Input: dimensioned drawing with shaded views. Units: mm. Origin: part minimum x, y, z. Give positions to 0.01 mm unless a question says otherwise; leave off trailing zeros. Write each loop counter-clockwise with the first axis right and the second up, starting at its lowest first coordinate (ties: lowest second). Pieces come first, ordered by that corner, then holes. Notation, with made-up numbers: (65.25, 14.25) -> (113.25, 14.25) arc R20 cw to (113.25, 24.25) -> close; hole circle Ø7 at (40.5, 59). An arc over 180 degrees is marked (long way). Answer as a JSON object with one key per item and string values. Group by question number.
(1) Section query A-A on x = 15. Output: boundary loops of the cut face in (y, z), plus the area to 3 significant figures.
(2) Section query B-B on y = 2.5. Output: boundary loops of the cut face in (x, z).
(3) Contact query for flat-ended pins moving along their axis: pin 1 Ø1.5 at (x, y) = (5.5, 0.5) entering from -Z; pin 2 Ø3 at (x, z) = (5, 15) entering from +Y; pin 3 Ø1.5 at (y, z) = (4, 8.5) entering from -X; pin 4 Ø2 at (x, y) = (4.5, 1.5) entering from +Z. Output: stop coordinate, or through.
(4) Material intervals for probe 1 along X at (y, z) = (1.7, 15); probe 2 along X at (y, z) = (1.95, 13.25), sorted ascending.
(5) Draft query along X for the marked faces 1, 2 and 3. Return one class per face: +X half, -X half, draft (parallel to the pull), parting line (faces both ways), or undercut.
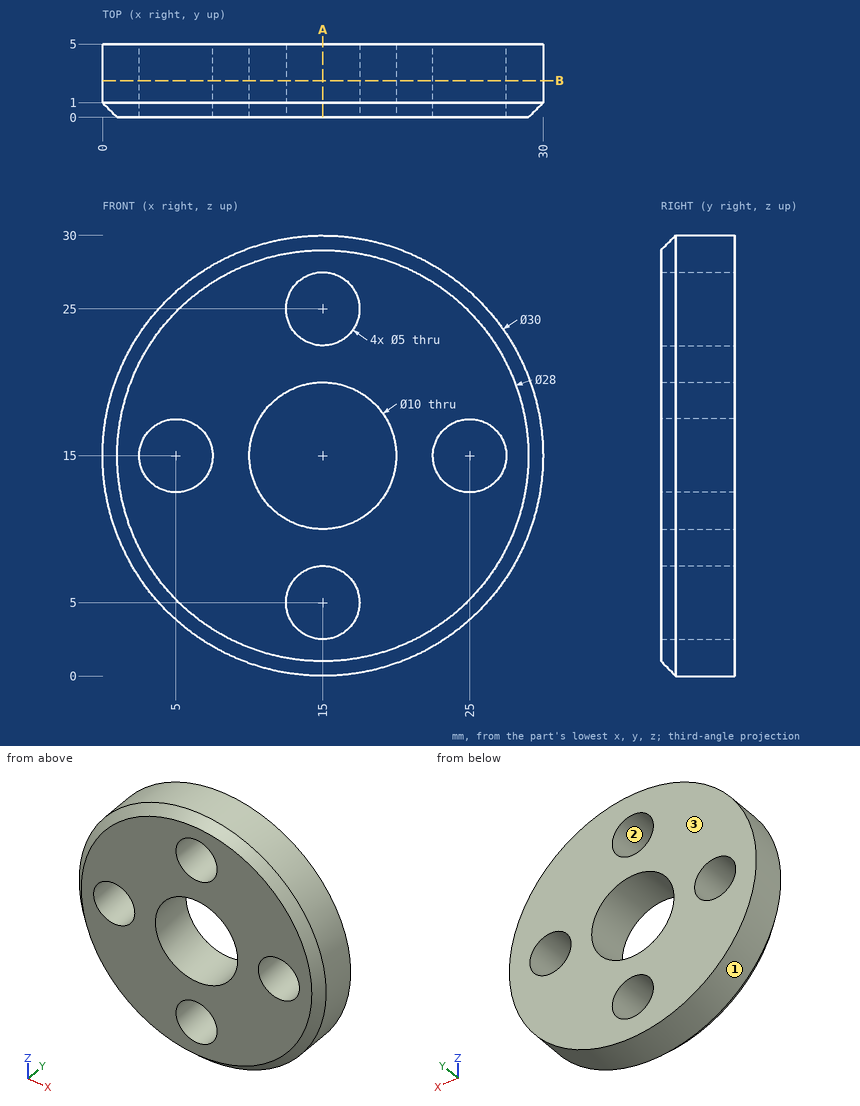
Answer list:
{
 "1": {"outline": "(0, 1) -> (1, 0) -> (5, 0) -> (5, 2.5) -> (0, 2.5) -> close; (0, 7.5) -> (5, 7.5) -> (5, 10) -> (0, 10) -> close; (0, 20) -> (5, 20) -> (5, 22.5) -> (0, 22.5) -> close; (0, 27.5) -> (5, 27.5) -> (5, 30) -> (1, 30) -> (0, 29) -> close", "area": "49.0 mm2"},
 "2": {"outline": "circle Ø30 at (15, 15); hole circle Ø5 at (5, 15); hole circle Ø10 at (15, 15); hole circle Ø5 at (15, 5); hole circle Ø5 at (15, 25); hole circle Ø5 at (25, 15)"},
 "3": {"pin 1": "z = 2.96", "pin 2": "through", "pin 3": "x = 1.15", "pin 4": "z = 26.61"},
 "4": {"probe 1": "0 to 2.5, 7.5 to 10, 20 to 22.5, 27.5 to 30", "probe 2": "0.1 to 3.21, 6.79 to 10.32, 19.68 to 23.21, 26.79 to 29.9"},
 "5": {"face 1": "parting line", "face 2": "undercut", "face 3": "draft"}
}
